Geometry check sheet. Reference: the model listing, model coordinates, mm. A direction names the side the tool comes from. Coordinates: 2 decimals unless noted, no trailing zeros. Order: outer loops, then holes, each group sorted by start corner. A loop starts at its lowest first (then second) coordinate and runs counter-clockwise, first axis right, second up. Notation, with made-up numbers: M 42.25,55.5 L 77.25,55.5 A24 ccw 77.25,69.5 Z; hole C -35,-26 d4. An arc over 180 degrees is marked long. One line per item, written item: value. Start each with the question number.
1) Access from +Z, -Z, +X, -X, +Y, -Y to the whole of each face (thin tool, end or side, straight path). Record for faces 5 (the flat face through (8, 3, -37)), 6 (the flat face through (4.5, 7.5, -36)), 7 (the flat face through (2, 0, -2)).
2) Sectioned sample at A-A, the plane y = 3. Enter the section's corners in (x, z).
3) Sectioned sample at B-B, the plane z = -27.5. Enter the section's corners in (x, y).
4) Draft check along Z on faces 1 (the cylindrical face through (2.475, 2.958, -31.785)), 2 (the flat face through (15, 0, -2)), 3 (the flat face through (-1, 8, -18)), 4 (the flat face through (8, 3, 2)). Enter one of: pulls with the +Z half, pulls with the -Z half, needs draft (parallel to the pull), parting line crosses it, or undercut.
5) Sectioned sample at D-D, the plane x = 14.75. Enter the section's corners in (y, z).
6) Go/stop test with flat-tipped pins: P1, Ø5, axis at x = 11.5, z = -13, coming from the +Y side; P2, Ø1.2, axis at x = 14.5, z = -32.5, coming from the +Y side. Record where each tip stops, or that it passes through.
7) Sectioned sample at C-C, the plane x = 9. Enter the section's corners in (y, z), then the cut area to 3 significant figures.
8) Thickness scan on L1, parallel to X at y = 0.25, z = -14; L2, parallel to X at y = 2.7, z = -32.5; L3, parallel to Z at x = 11.5, y = 3. Record the ranges inside material, lowest first. Write a range as from..to.
```python
from build123d import *

# Parameters (mm, degrees)
SKETCH1_W           = 21
SKETCH1_H           = 39
SKETCH1_W_2         = 17
SKETCH1_H_2         = 35
BOSS_EXTRUDE1_DEPTH = 8
SKETCH2_W           = 21
SKETCH2_H           = 39
BOSS_EXTRUDE2_DEPTH = 2
SKETCH3_R           = 0.75
BOSS_EXTRUDE3_DEPTH = 6
CUT_EXTRUDE1_REACH  = 46.113
SKETCH4_W           = 8
SKETCH4_H           = 1


with BuildPart() as part:
    # Sketch1 → Boss-Extrude1 (new body)
    with BuildSketch(Plane(origin=(0, 0, 0), x_dir=(1, 0, 0), z_dir=(0, 1, 0))):
        with Locations((8.5, 17.5)):
            Rectangle(SKETCH1_W, SKETCH1_H)
        with Locations((8.5, 17.5)):
            Rectangle(SKETCH1_W_2, SKETCH1_H_2, mode=Mode.SUBTRACT)
    extrude(amount=BOSS_EXTRUDE1_DEPTH)

    # Sketch2 → Boss-Extrude2 (add)
    with BuildSketch(Plane.XZ):
        with Locations((8.5, -17.5)):
            Rectangle(SKETCH2_W, SKETCH2_H)
    extrude(amount=BOSS_EXTRUDE2_DEPTH)

    # Sketch3 → Boss-Extrude3 (add)
    # profile 1 of 4: a face of its own
    with BuildSketch(Plane(origin=(0, 0, 0), x_dir=(1, 0, 0), z_dir=(0, 1, 0))):
        with BuildLine():
            Line((0, 30), (0, 35))
            Line((0, 35), (5, 35))
            ThreePointArc((5, 35), (3.535533906, 31.464466094), (0, 30))
        make_face()
        with Locations(Location((2.25, 32.5, 0), (0, 0, 270))):
            Circle(SKETCH3_R, mode=Mode.SUBTRACT)
    # profile 2 of 4: a face of its own
    with BuildSketch(Plane(origin=(0, 0, 0), x_dir=(1, 0, 0), z_dir=(0, 1, 0))):
        with BuildLine():
            Line((17, 0), (12, 0))
            ThreePointArc((12, 0), (13.464466094, 3.535533906), (17, 5))
            Line((17, 5), (17, 0))
        make_face()
        with Locations(Location((14.75, 2.5, 0), (0, 0, 270))):
            Circle(SKETCH3_R, mode=Mode.SUBTRACT)
    # profile 3 of 4: a face of its own
    with BuildSketch(Plane(origin=(0, 0, 0), x_dir=(1, 0, 0), z_dir=(0, 1, 0))):
        with BuildLine():
            Line((17, 35), (12, 35))
            ThreePointArc((12, 35), (13.464466094, 31.464466094), (17, 30))
            Line((17, 30), (17, 35))
        make_face()
        with Locations(Location((14.75, 32.5, 0), (0, 0, 270))):
            Circle(SKETCH3_R, mode=Mode.SUBTRACT)
    # profile 4 of 4: a face of its own
    with BuildSketch(Plane(origin=(0, 0, 0), x_dir=(1, 0, 0), z_dir=(0, 1, 0))):
        with BuildLine():
            Line((0, 0), (0, 5))
            ThreePointArc((0, 5), (3.535533906, 3.535533906), (5, 0))
            Line((5, 0), (0, 0))
        make_face()
        with Locations(Location((2.25, 2.5, 0), (0, 0, 270))):
            Circle(SKETCH3_R, mode=Mode.SUBTRACT)
    extrude(amount=BOSS_EXTRUDE3_DEPTH)

    # Sketch4 → Cut-Extrude1 (cut, up to next)
    with BuildSketch(Plane(origin=(0, 0, -37), x_dir=(-1, 0, 0), z_dir=(0, 0, -1)), mode=Mode.PRIVATE) as cut_extrude1_sk1:
        with Locations((-8.5, 7.5)):
            Rectangle(SKETCH4_W, SKETCH4_H)
    cut_extrude1_tool1 = extrude(cut_extrude1_sk1.sketch, amount=-CUT_EXTRUDE1_REACH, mode=Mode.PRIVATE) & part.part
    add(cut_extrude1_tool1.solids().sort_by_distance((8.5, 7.5, -37))[0], mode=Mode.SUBTRACT)


solid = part.part
```
Final values:
1. face 5: -Z, +X, -X, +Y, -Y
1. face 6: -Z, +Y
1. face 7: +Y
2. outline: M -2,-37 L 19,-37 L 19,2 L -2,2 Z; hole M 0,-30 A5 cw 5,-35 L 12,-35 A5 cw 17,-30 L 17,-5 A5 cw 12,0 L 5,0 A5 cw 0,-5 Z; hole C 2.25,-32.5 d1.5; hole C 2.25,-2.5 d1.5; hole C 14.75,-32.5 d1.5; hole C 14.75,-2.5 d1.5
3. outline: M -2,-2 L 19,-2 L 19,8 L 17,8 L 17,0 L 0,0 L 0,8 L -2,8 Z
4. face 1: undercut
4. face 2: undercut
4. face 3: needs draft
4. face 4: pulls with the +Z half
5. outline: M -2,-37 L 8,-37 L 8,-35 L 6,-35 L 6,-33.25 L 0,-33.25 L 0,-31.75 L 6,-31.75 L 6,-30.53 L 0,-30.53 L 0,-4.47 L 6,-4.47 L 6,-3.25 L 0,-3.25 L 0,-1.75 L 6,-1.75 L 6,0 L 8,0 L 8,2 L -2,2 Z
6. P1: stops at y = 0
6. P2: stops at y = 6
7. outline: M -2,-37 L 7,-37 L 7,-35 L 0,-35 L 0,0 L 8,0 L 8,2 L -2,2 Z
7. area: 108 mm^2
8. L1: x = -2..0, 17..19
8. L2: x = -2..1.5, 3..4.33, 12.67..14, 15.5..19
8. L3: z = -37..-35, 0..2
